Source: CAD feature listing. Evaluate the final solid. Frame: model axes, mm. A direction names the side the tool comes from. Give positions to 0.01 mm unless a question says otherwise; leave off trailing zeros. Order: outer loops, then holes, each group sorted by start corner. A loop starts at its lowest first (then second) coordinate and runs counter-clockwise, first axis right, second up.
from build123d import *

# Parameters (mm, degrees)
F1_DEPTH = 100
F2_R     = 2
F3_DEPTH = 72
F4_R     = 2
F4_R_2   = 1.5
F5_DEPTH = 6.5


with BuildPart() as f1:
    # F0 (on Top) → F1 (new body)
    with BuildSketch(Plane.XY):
        with BuildLine():
            ThreePointArc((0, 0.5), (0.146447, 0.146447), (0.5, 0))
            Line((0.5, 0), (94.5, 0))
            ThreePointArc((94.5, 0), (94.853553, 0.146447), (95, 0.5))
            Line((95, 0.5), (95, 6))
            ThreePointArc((95, 6), (94.853553, 6.353553), (94.5, 6.5))
            Line((94.5, 6.5), (84, 6.5))
            ThreePointArc((84, 6.5), (83.646447, 6.646447), (83.5, 7))
            Line((83.5, 7), (83.5, 46))
            ThreePointArc((83.5, 46), (83.353553, 46.353553), (83, 46.5))
            Line((83, 46.5), (79, 46.5))
            ThreePointArc((79, 46.5), (78.646447, 46.353553), (78.5, 46))
            Line((78.5, 46), (78.5, 7))
            ThreePointArc((78.5, 7), (78.353553, 6.646447), (78, 6.5))
            Line((78, 6.5), (17, 6.5))
            ThreePointArc((17, 6.5), (16.646447, 6.646447), (16.5, 7))
            Line((16.5, 7), (16.5, 46))
            ThreePointArc((16.5, 46), (16.353553, 46.353553), (16, 46.5))
            Line((16, 46.5), (12, 46.5))
            ThreePointArc((12, 46.5), (11.646447, 46.353553), (11.5, 46))
            Line((11.5, 46), (11.5, 7))
            ThreePointArc((11.5, 7), (11.353553, 6.646447), (11, 6.5))
            Line((11, 6.5), (0.5, 6.5))
            ThreePointArc((0.5, 6.5), (0.146447, 6.353553), (0, 6))
            Line((0, 6), (0, 0.5))
        make_face()
    extrude(amount=F1_DEPTH)

    # F2 (on face) → F3 (cut, through all)
    with BuildSketch(Plane.YZ.offset(83.5)):
        with Locations((37.5, 80)):
            Circle(F2_R)
        with Locations((37.5, 60)):
            Circle(F2_R)
        with Locations((37.5, 40)):
            Circle(F2_R)
        with Locations((37.5, 20)):
            Circle(F2_R)
    extrude(amount=-F3_DEPTH, mode=Mode.SUBTRACT)

    # F4 (on face) → F5 (cut, through all)
    with BuildSketch(Plane(origin=(0, 6.5, 0), x_dir=(-1, 0, 0), z_dir=(0, 1, 0))):
        with Locations((-47.5, 80)):
            Circle(F4_R)
        with Locations((-47.5, 60)):
            Circle(F4_R)
        with Locations((-47.5, 40)):
            Circle(F4_R)
        with Locations((-47.5, 20)):
            Circle(F4_R)
        with Locations((-5.5, 80)):
            Circle(F4_R_2)
        with Locations((-5.5, 20)):
            Circle(F4_R_2)
        with Locations((-89.5, 80)):
            Circle(F4_R_2)
        with Locations((-89.5, 20)):
            Circle(F4_R_2)
    extrude(amount=-F5_DEPTH, mode=Mode.SUBTRACT)


solid = f1.part
1) Ray query, L1, parallel to Z at x = 47.5, y = 5; L2, parallel to Z at x = 89.5, y = 3.5; L3, parallel to X at y = 10, z = 79.5. Return the intervals inside material, ascending.
Checks:
L1: z = 0 to 18, 22 to 38, 42 to 58, 62 to 78, 82 to 100
L2: z = 0 to 18.5, 21.5 to 78.5, 81.5 to 100
L3: x = 11.5 to 16.5, 78.5 to 83.5
2) Reachability of faces 1 (the face through (11.5, 27, 49)), 2 (the face through (89, 6.5, 49)), 3 (the face through (78.5, 27, 49)) from +Z, -Z, +X, -X, +Y, -Y: full face, straight path, thin tool, end or side. Return the list, or none.
Checks:
face 1: +Z, -Z, -X, +Y
face 2: +Z, -Z, +X, +Y
face 3: +Z, -Z, +Y
3) Pull-direction query (Z, two-part tool) for faces 4 (the face through (14.035, 37.24, 81.983)), 5 (the face through (51, 6, 0)), 6 (the face through (6, 6.5, 49)); classes: +Z half, -Z half, draft (parallel to the pull), parting line (faces both ways), or undercut.
Checks:
face 4: undercut
face 5: -Z half
face 6: draft
4) Section query A-A on y = 23. Output: boundary loops of the cut face in (x, z).
Checks:
outline: (11.5, 0) - (16.5, 0) - (16.5, 100) - (11.5, 100) - close; (78.5, 0) - (83.5, 0) - (83.5, 100) - (78.5, 100) - close
5) First-contact query: pin 1 Ø5 at (x, z) = (29, 89) entering from +Y; pin 2 Ø5 at (y, z) = (37.5, 20) entering from -X; pin 3 Ø11.5 at (y, z) = (27, 69.5) entering from +X. Flat tips, straight axial feed; report the tip coordinate or a pass-through.
Checks:
pin 1: stops at y = 6.5
pin 2: stops at x = 11.5
pin 3: stops at x = 83.5
6) Section query C-C on x = 47.5. Output: boundary loops of the cut face in (y, z).
Checks:
outline: (0, 0) - (6.5, 0) - (6.5, 18) - (0, 18) - close; (0, 22) - (6.5, 22) - (6.5, 38) - (0, 38) - close; (0, 42) - (6.5, 42) - (6.5, 58) - (0, 58) - close; (0, 62) - (6.5, 62) - (6.5, 78) - (0, 78) - close; (0, 82) - (6.5, 82) - (6.5, 100) - (0, 100) - close
7) Section query B-B on x = 5.5. Output: boundary loops of the cut face in (y, z), and give its area (3 significant figures).
Checks:
outline: (0, 0) - (6.5, 0) - (6.5, 18.5) - (0, 18.5) - close; (0, 21.5) - (6.5, 21.5) - (6.5, 78.5) - (0, 78.5) - close; (0, 81.5) - (6.5, 81.5) - (6.5, 100) - (0, 100) - close
area: 611 mm2
8) Section query D-D on z = 30. Output: boundary loops of the cut face in (x, y), and give its area (3 significant figures).
Checks:
outline: (0, 0.5) arc R0.5 ccw to (0.5, 0) - (94.5, 0) arc R0.5 ccw to (95, 0.5) - (95, 6) arc R0.5 ccw to (94.5, 6.5) - (84, 6.5) arc R0.5 cw to (83.5, 7) - (83.5, 46) arc R0.5 ccw to (83, 46.5) - (79, 46.5) arc R0.5 ccw to (78.5, 46) - (78.5, 7) arc R0.5 cw to (78, 6.5) - (17, 6.5) arc R0.5 cw to (16.5, 7) - (16.5, 46) arc R0.5 ccw to (16, 46.5) - (12, 46.5) arc R0.5 ccw to (11.5, 46) - (11.5, 7) arc R0.5 cw to (11, 6.5) - (0.5, 6.5) arc R0.5 ccw to (0, 6) - close
area: 1,020 mm2
